Input: part model. Units: mm. Frame: model coordinates. A direction names the side the tool comes from. Coordinates: 2 decimals unless noted, no trailing zeros. Loops run counter-clockwise (first coordinate to the right, second up) from the corner with the lowest first, then second, coordinate; pieces in that order, holes last. Notation, with made-up numbers: (-36.5, 44.25) -> (4.5, 44.25) arc R32 ccw to (4.5, 80.25) -> close; hole circle Ø8 at (-10, -12). An arc over 180 degrees is marked (long way). Answer as a JSON object with one key per item and string values.
from build123d import *

# Parameters (mm, degrees)
BOSS_EXTRUDE1_DEPTH            = 6
SKETCH3_R                      = 1.75
CUT_EXTRUDE2_DEPTH             = 69.176242196
BOSS_EXTRUDE2_DEPTH            = 13
BOSS_EXTRUDE3_DEPTH            = 6
CUT_EXTRUDE3_REACH             = 74.367
SKETCH6_R                      = 1.75
CUT_EXTRUDE4_REACH             = 74.367
SKETCH8_R                      = 15.1
BOSS_EXTRUDE4_DEPTH            = 11
SKETCH9_R                      = 1.75
CUT_EXTRUDE5_DEPTH             = 10
CUT_EXTRUDE6_REACH             = 78.864
SKETCH11_R                     = 3
CUT_EXTRUDE6_DIRECTION_2_DEPTH = 77.863515556
CUT_EXTRUDE7_REACH             = 74.719
SKETCH12_R                     = 3


with BuildPart() as part:
    # Sketch1 → Boss-Extrude1 (new body)
    with BuildSketch(Plane(origin=(0, 0, 0), x_dir=(1, 0, 0), z_dir=(0, 1, 0))):
        with BuildLine():
            Line((-50, 16), (50, 16))
            ThreePointArc((50, 16), (66, 0), (50, -16))
            Line((50, -16), (-50, -16))
            ThreePointArc((-50, -16), (-66, 0), (-50, 16))
        make_face()
    extrude(amount=BOSS_EXTRUDE1_DEPTH)

    # Sketch3 → Cut-Extrude2 (cut, through all)
    with BuildSketch(Plane.XZ):
        with Locations(Location((50, 0, 0), (0, 0, 270))):
            Circle(SKETCH3_R)
    extrude(amount=-CUT_EXTRUDE2_DEPTH, mode=Mode.SUBTRACT)

    # Sketch4 → Boss-Extrude2 (add)
    with BuildSketch(Plane(origin=(0, 6, 0), x_dir=(1, 0, 0), z_dir=(0, 1, 0))):
        with BuildLine():
            Line((-50, 16), (30, 16))
            add(Edge.make_bspline(
                [(30, 16), (21.992860017, -10.862158013), (-23.676278326, 6.118145935), (-34.285676412, -16)],
                knots=[0, 0, 0, 0, 1, 1, 1, 1], degree=3))
            Line((-34.285676412, -16), (-50, -16))
            ThreePointArc((-50, -16), (-66, 0), (-50, 16))
        make_face()
    extrude(amount=BOSS_EXTRUDE2_DEPTH)

    # Sketch5 → Boss-Extrude3 (add)
    with BuildSketch(Plane(origin=(0, 19, 0), x_dir=(1, 0, 0), z_dir=(0, 1, 0))):
        with BuildLine():
            Line((-50, 16), (50, 16))
            ThreePointArc((50, 16), (66, 0), (50, -16))
            Line((50, -16), (-50, -16))
            ThreePointArc((-50, -16), (-66, 0), (-50, 16))
        make_face()
    extrude(amount=BOSS_EXTRUDE3_DEPTH)

    # Sketch6 → Cut-Extrude3 (cut, up to next)
    with BuildSketch(Plane(origin=(0, 25, 0), x_dir=(1, 0, 0), z_dir=(0, 1, 0)), mode=Mode.PRIVATE) as cut_extrude3_sk1:
        with Locations(Location((50, 0, 0), (0, 0, 90))):
            Circle(SKETCH6_R)
    cut_extrude3_tool1 = extrude(cut_extrude3_sk1.sketch, amount=-CUT_EXTRUDE3_REACH, mode=Mode.PRIVATE) & part.part
    add(cut_extrude3_tool1.solids().sort_by_distance((50, 25, 0))[0], mode=Mode.SUBTRACT)

    # Sketch7 → Cut-Extrude4 (cut, up to next)
    with BuildSketch(Plane(origin=(0, 25, 0), x_dir=(1, 0, 0), z_dir=(0, 1, 0)), mode=Mode.PRIVATE) as cut_extrude4_sk1:
        with BuildLine():
            ThreePointArc((-37.731263809, -10.270253759), (-43.22962557, -14.496966237), (-50, -16))
            Line((-50, -16), (50, -16))
            add(Edge.make_bspline(
                [(-37.731263809, -10.270253759), (-30.332556703, -1.431836739), (6.050402888, -3.364587973), (38.512231583, -16), (50, -16)],
                knots=[0, 0, 0, 0, 0.426660683, 1, 1, 1, 1], degree=3))
        make_face()
    cut_extrude4_tool1 = extrude(cut_extrude4_sk1.sketch, amount=-CUT_EXTRUDE4_REACH, mode=Mode.PRIVATE) & part.part
    add(cut_extrude4_tool1.solids().sort_by_distance((-6.915299, 25, 11.013102))[0], mode=Mode.SUBTRACT)

    # Sketch8 → Boss-Extrude4 (add)
    with BuildSketch(Plane.XZ):
        with Locations(Location((-50, 0, 0), (0, 0, 90))):
            Circle(SKETCH8_R)
    extrude(amount=BOSS_EXTRUDE4_DEPTH)

    # Sketch9 → Cut-Extrude5 (cut)
    with BuildSketch(Plane.XZ.offset(11)):
        with Locations(Location((-50, 6.75, 0), (0, 0, 270))):
            Circle(SKETCH9_R)
        with Locations(Location((-50, -6.75, 0), (0, 0, 270))):
            Circle(SKETCH9_R)
    extrude(amount=-CUT_EXTRUDE5_DEPTH, mode=Mode.SUBTRACT)

    # Sketch11 → Cut-Extrude6 (cut, up to next)
    with BuildSketch(Plane.XZ.offset(11), mode=Mode.PRIVATE) as cut_extrude6_sk1:
        with Locations(Location((-50, 0, 0), (0, 0, 90))):
            Circle(SKETCH11_R)
    cut_extrude6_tool1 = extrude(cut_extrude6_sk1.sketch, amount=-CUT_EXTRUDE6_REACH, mode=Mode.PRIVATE) & part.part
    add(cut_extrude6_tool1.solids().sort_by_distance((-50, -11, 0))[0], mode=Mode.SUBTRACT)

    # Sketch11 → Cut-Extrude6 direction 2 (cut)
    with BuildSketch(Plane.XZ.offset(11)):
        with Locations(Location((-50, 0, 0), (0, 0, 90))):
            Circle(SKETCH11_R)
    extrude(amount=CUT_EXTRUDE6_DIRECTION_2_DEPTH, mode=Mode.SUBTRACT)

    # Sketch12 → Cut-Extrude7 (cut, up to next)
    with BuildSketch(Plane.XZ.offset(1), mode=Mode.PRIVATE) as cut_extrude7_sk1:
        with Locations(Location((-50, 6.75, 0), (0, 0, 270))):
            Circle(SKETCH12_R)
    cut_extrude7_tool1 = extrude(cut_extrude7_sk1.sketch, amount=-CUT_EXTRUDE7_REACH, mode=Mode.PRIVATE) & part.part
    # Sketch12 → Cut-Extrude7 (cut, up to next)
    with BuildSketch(Plane.XZ.offset(1), mode=Mode.PRIVATE) as cut_extrude7_sk2:
        with Locations(Location((-50, -6.75, 0), (0, 0, 270))):
            Circle(SKETCH12_R)
    cut_extrude7_tool2 = extrude(cut_extrude7_sk2.sketch, amount=-CUT_EXTRUDE7_REACH, mode=Mode.PRIVATE) & part.part
    add(cut_extrude7_tool1.solids().sort_by_distance((-50, -1, 6.75))[0], mode=Mode.SUBTRACT)
    add(cut_extrude7_tool2.solids().sort_by_distance((-50, -1, -6.75))[0], mode=Mode.SUBTRACT)


solid = part.part
1. Pin query (flat end, axial travel): P1, Ø5, axis at y = -1, z = -3.5, coming from the +X side; P2, Ø3, axis at x = -50.5, z = -6, coming from the +Y side; P3, Ø10, axis at y = 17, z = -10.5, coming from the -X side (3 decimals). Return the tip coordinate at first contact, or that it passes through.
Reply:
{"P1": "stops at x = 65.95", "P2": "stops at y = -1", "P3": "stops at x = -65.025"}
2. Access query for faces 1 (the face through (-51.71, -6.07, -6.37)), 2 (the face through (-47.47, 11.82, 5.14)), 3 (the face through (-64.97, -5.42, -1.97)). Directions: +Z, -Z, +X, -X, +Y, -Y. A direction counts if a zero-diameter tool reaches every point of the face in a straight line with its end or side. Return the directions, or none.
Reply:
{"face 1": "+Y, -Y", "face 2": "+Y", "face 3": "-Y"}
3. Line query: line 1 along Y through (x, z) = (27, -9.5); line 2 along Y through (x, z) = (-0.5, -7.5); line 3 along X through (y, z) = (-10, 0). Output: solid intervals per line, ascending.
Reply:
{"line 1": "y = 0 to 6, 19 to 25", "line 2": "y = 0 to 25", "line 3": "x = -65.1 to -53, -47 to -34.9"}
4. Section query A-A (x = 55.5). Return loops of the section in (y, z).
Reply:
{"outline": "(0, -15.02) -> (6, -15.02) -> (6, 15.02) -> (0, 15.02) -> close; (19, -15.02) -> (25, -15.02) -> (25, 15.02) -> (19, 15.02) -> close"}
5. Mould query, pull axis Y, two halves, no side actions, for faces 4 (the face through (36, 6, 0)), 5 (the face through (-52, -1, -7)), 6 (the face through (36, 19, 0)), 7 (the face through (51.71, 22.04, 0.38)). Classes: pulls with the +Y half, pulls with the -Y half, needs draft (parallel to the pull), parting line crosses it, or undercut.
Reply:
{"face 4": "undercut", "face 5": "pulls with the +Y half", "face 6": "undercut", "face 7": "needs draft"}
6. Section query C-C (z = 0). Count the separate pieces of the cut face and the enclosed holes in it, plus the area to 3 significant figures.
Reply:
{"separate pieces": "4", "enclosed holes": "0", "area": "2,640 mm2"}
7. Section query B-B (y = -3). Return loops of the section in (x, z).
Reply:
{"outline": "circle Ø30.2 at (-50, 0); hole circle Ø6 at (-50, 0); hole circle Ø3.5 at (-50, -6.75); hole circle Ø3.5 at (-50, 6.75)"}
